Design review of the part built by this model. Coordinates are the model's own, in mm. A direction names the side the tool comes from. Coordinates: 2 decimals unless noted, no trailing zeros. Order: outer loops, then holes, each group sorted by start corner. A loop starts at its lowest first (then second) coordinate and runs counter-clockwise, first axis right, second up. Notation, with made-up numbers: (51.5, 7) -> (79.5, 7) arc R18 ccw to (79.5, 18) -> close; hole circle Ø1 at (-35, -7). An arc over 180 degrees is marked (long way). Use a Markdown table: item, result. Add a question column.
Q1. Wall thickness on probe 1 along Y at (x, z) = (-9, 5.5); probe 2 along Y at (x, z) = (12.5, 18.5); probe 3 along X at (y, z) = (-19, 9): over which ranges is each line inside the solid? List them lowest first.
Q2. Insertion check: pin 1 (11 mm diameter, centred on x = 13, z = 14.5, fed in from +Y); pin 2 (9.5 mm diameter, centred on y = -12.5, z = 11, fed in from -X); pin 3 (4 mm diameter, centred on y = -1, z = 14, fed in from +X). Each pin has a flat end and moves straight along its axis. Give the tip position at first contact, or say it passes through.
Q3. Add section A-A (z = 10.25). State the section outline as (x, y) points.
Q4. The part is to be moulded in two halves that separate along Y. For faces 4 (the face through (22.1, -13, 15)), 5 (the face through (-20, -13, 11)), 6 (the face through (-13, -8, 21)), 7 (the face through (-13, 22.5, 15)), say which applies: pulls with the +Y half, pulls with the -Y half, needs draft (parallel to the pull), parting line crosses it, or undercut.
Q5. Add section B-B (y = -15). State the section outline as (x, z) points.
Q6. Add section C-C (z = 21). State the section outline as (x, y) points, then the cut area to 3 significant figures.
Q7. Add section D-D (x = 12.5). State the section outline as (y, z) points, then the cut area to 3 significant figures.
Q8. Machinability: for faces 1 (the face through (-13, -17, 21)), 2 (the face through (22.5, -13, 15)), 3 (the face through (12, -7.5, 15)), which of the approach directions +Z, -Z, +X, -X, +Y, -Y give a long, thin tool a straight path to every point of the face, cutting with its end or side? Answer none if there is none.
from build123d import *

# Parameters (mm, degrees)
F0_W     = 50
F0_H     = 50
F0_W_2   = 15
F0_H_2   = 15
F0_W_3   = 20
F0_H_3   = 20
F0_R     = 10.5
F0_W_4   = 19.04
F0_H_4   = 19.04
F0_W_5   = 19.2
F0_H_5   = 19.2
F0_W_6   = 10
F0_H_6   = 10
F0_R_2   = 7.5
F1_DEPTH = 5
F2_DEPTH = 25
F3_DEPTH = 25
F4_DEPTH = 25
F5_DEPTH = 25
F6_R     = 1
F7_SIZE  = 7


with BuildPart() as f1:
    # F0 (on Top) → F1 (new body)
    with BuildSketch(Plane.XY):
        Rectangle(F0_W, F0_H)
        with Locations((-12.5, -12.5)):
            Rectangle(F0_W_2, F0_H_2, mode=Mode.SUBTRACT)
        with Locations((12.5, -12.5)):
            Rectangle(F0_W_3, F0_H_3, mode=Mode.SUBTRACT)
        with Locations((-12.5, 12.500000177)):
            Rectangle(F0_W_3, F0_H_3, mode=Mode.SUBTRACT)
        with Locations((12.5, 12.500000177)):
            Circle(F0_R, mode=Mode.SUBTRACT)
        with Locations((-12.5, 12.500000177)):
            Rectangle(F0_W_3, F0_H_3)
        with Locations((-12.5, 12.500000177)):
            Rectangle(F0_W_4, F0_H_4, mode=Mode.SUBTRACT)
        with Locations((12.5, -12.5)):
            Rectangle(F0_W_3, F0_H_3)
        with Locations((12.5, -12.5)):
            Rectangle(F0_W_5, F0_H_5, mode=Mode.SUBTRACT)
        with Locations((12.5, -12.5)):
            Rectangle(F0_W_5, F0_H_5)
        with Locations((12.5, -12.5)):
            Rectangle(F0_W_6, F0_H_6, mode=Mode.SUBTRACT)
        with Locations((-12.5, 12.500000177)):
            Rectangle(F0_W_4, F0_H_4)
        with Locations((12.5, 12.500000177)):
            Circle(F0_R)
        with Locations((12.5, 12.500000177)):
            Circle(F0_R_2, mode=Mode.SUBTRACT)
        with Locations((-12.5, -12.5)):
            Rectangle(F0_W_2, F0_H_2)
        with Locations((12.5, 12.500000177)):
            Circle(F0_R_2)
        with Locations((12.5, -12.5)):
            Rectangle(F0_W_6, F0_H_6)
    extrude(amount=F1_DEPTH)

    # F0 (on Top) → F2 (join)
    with BuildSketch(Plane.XY):
        with Locations((-12.5, 12.500000177)):
            Rectangle(F0_W_3, F0_H_3)
        with Locations((-12.5, 12.500000177)):
            Rectangle(F0_W_4, F0_H_4, mode=Mode.SUBTRACT)
    extrude(amount=F2_DEPTH)

    # F0 (on Top) → F3 (join)
    with BuildSketch(Plane.XY):
        with Locations((12.5, -12.5)):
            Rectangle(F0_W_3, F0_H_3)
        with Locations((12.5, -12.5)):
            Rectangle(F0_W_5, F0_H_5, mode=Mode.SUBTRACT)
        with Locations((12.5, -12.5)):
            Rectangle(F0_W_6, F0_H_6)
    extrude(amount=F3_DEPTH)

    # F0 (on Top) → F4 (join)
    with BuildSketch(Plane.XY):
        with Locations((-12.5, -12.5)):
            Rectangle(F0_W_2, F0_H_2)
    extrude(amount=F4_DEPTH)

    # F0 (on Top) → F5 (join)
    with BuildSketch(Plane.XY):
        with Locations((12.5, 12.500000177)):
            Circle(F0_R)
        with Locations((12.5, 12.500000177)):
            Circle(F0_R_2, mode=Mode.SUBTRACT)
    extrude(amount=F5_DEPTH)

    # F6
    f6_edges = [f1.edges().sort_by_distance(p)[0] for p in [
        (-25, -25, 2.5),
        (2, 12.5, 25),
        (5, 12.5, 25),
    ]]
    fillet(f6_edges, radius=F6_R)

    # F7
    f7_edges = [f1.edges().sort_by_distance(p)[0] for p in [
        (-12.5, -5, 25),
        (-20, -12.5, 25),
        (-12.5, -20, 25),
        (-5, -12.5, 25),
    ]]
    chamfer(f7_edges, length=F7_SIZE)


solid = f1.part
Established:
| question | item | result |
|---|---|---|
| 1 | probe 1 | -20 to -5, 2.5 to 2.98, 22.02 to 22.5 |
| 1 | probe 2 | -22.5 to -22.1, -17.5 to -7.5, -2.9 to -2.5, 2 to 5, 20 to 23 |
| 1 | probe 3 | -20 to -5, 2.5 to 2.9, 22.1 to 22.5 |
| 2 | pin 1 | y = 23 |
| 2 | pin 2 | x = -20 |
| 2 | pin 3 | x = 22.5 |
| 3 | outline | (-22.5, 2.5) -> (-2.5, 2.5) -> (-2.5, 22.5) -> (-22.5, 22.5) -> close; (-20, -20) -> (-5, -20) -> (-5, -5) -> (-20, -5) -> close; circle Ø21 at (12.5, 12.5); (2.5, -22.5) -> (22.5, -22.5) -> (22.5, -2.5) -> (2.5, -2.5) -> close; (7.5, -17.5) -> (17.5, -17.5) -> (17.5, -7.5) -> (7.5, -7.5) -> close; hole (-22.02, 2.98) -> (-2.98, 2.98) -> (-2.98, 22.02) -> (-22.02, 22.02) -> close; hole (2.9, -22.1) -> (22.1, -22.1) -> (22.1, -2.9) -> (2.9, -2.9) -> close; hole circle Ø15 at (12.5, 12.5) |
| 4 | face 4 | undercut |
| 4 | face 5 | needs draft |
| 4 | face 6 | undercut |
| 4 | face 7 | pulls with the +Y half |
| 5 | outline | (-25, 0) -> (25, 0) -> (25, 5) -> (22.5, 5) -> (22.5, 25) -> (22.1, 25) -> (22.1, 5) -> (17.5, 5) -> (17.5, 25) -> (7.5, 25) -> (7.5, 5) -> (2.9, 5) -> (2.9, 25) -> (2.5, 25) -> (2.5, 5) -> (-5, 5) -> (-5, 18) -> (-10, 23) -> (-15, 23) -> (-20, 18) -> (-20, 5) -> (-25, 5) -> close |
| 6 | outline | (-22.5, 2.5) -> (-2.5, 2.5) -> (-2.5, 22.5) -> (-22.5, 22.5) -> close; (-17, -17) -> (-8, -17) -> (-8, -8) -> (-17, -8) -> close; circle Ø21 at (12.5, 12.5); (2.5, -22.5) -> (22.5, -22.5) -> (22.5, -2.5) -> (2.5, -2.5) -> close; (7.5, -17.5) -> (17.5, -17.5) -> (17.5, -7.5) -> (7.5, -7.5) -> close; hole (-22.02, 2.98) -> (-2.98, 2.98) -> (-2.98, 22.02) -> (-22.02, 22.02) -> close; hole (2.9, -22.1) -> (22.1, -22.1) -> (22.1, -2.9) -> (2.9, -2.9) -> close; hole circle Ø15 at (12.5, 12.5) |
| 6 | area | 419 mm^2 |
| 7 | outline | (-25, 0) -> (25, 0) -> (25, 5) -> (23, 5) -> (23, 24) arc R1 ccw to (22, 25) -> (21, 25) arc R1 ccw to (20, 24) -> (20, 5) -> (5, 5) -> (5, 24) arc R1 ccw to (4, 25) -> (3, 25) arc R1 ccw to (2, 24) -> (2, 5) -> (-2.5, 5) -> (-2.5, 25) -> (-2.9, 25) -> (-2.9, 5) -> (-7.5, 5) -> (-7.5, 25) -> (-17.5, 25) -> (-17.5, 5) -> (-22.1, 5) -> (-22.1, 25) -> (-22.5, 25) -> (-22.5, 5) -> (-25, 5) -> close |
| 7 | area | 585 mm^2 |
| 8 | face 1 | +Z, -X, -Y |
| 8 | face 2 | +Z, +X, -Y |
| 8 | face 3 | +Z |
